```python
from build123d import *

# Parameters (mm, degrees)
SKETCH1_R                = 52.5
BOSS_EXTRUDE1_DEPTH      = 2
SKETCH2_R                = 52.5
SKETCH2_R_2              = 50.25
BOSS_EXTRUDE2_DEPTH      = 100
BOSS_EXTRUDE3_DEPTH      = 90
BOSS_EXTRUDE3_DEPTH_BACK = 15
BOSS_EXTRUDE4_DEPTH      = 15
BOSS_EXTRUDE4_DEPTH_BACK = 10
SKETCH7_R                = 15
SKETCH8_R                = 37.5
BOSS_EXTRUDE5_DEPTH      = 5
SKETCH9_R                = 1.5
CUT_EXTRUDE1_DEPTH       = 6
CUT_EXTRUDE2_DEPTH       = 265.804278799
CUT_EXTRUDE2_DEPTH_BACK  = 265.804278799
SKETCH5_R                = 4.5
CUT_EXTRUDE3_START       = -4
CUT_EXTRUDE3_DEPTH       = 20
CUT_EXTRUDE4_START       = -3
SKETCH11_W               = 8
SKETCH11_H               = 15
CUT_EXTRUDE4_DEPTH       = 95
SKETCH12_R               = 3
CUT_EXTRUDE5_DEPTH       = 20
SKETCH13_R               = 3.5
SKETCH13_R_2             = 3
BOSS_EXTRUDE6_DEPTH      = 6.5
CHAMFER1_SIZE            = 0.5
SKETCH14_R               = 51.5
CUT_EXTRUDE6_DEPTH       = 48
SKETCH15_R               = 1.5
BOSS_EXTRUDE7_DEPTH      = 5
BOSS_EXTRUDE8_DEPTH      = 5
BOSS_EXTRUDE9_DEPTH      = 6
BOSS_EXTRUDE9_DEPTH_BACK = 6
SKETCH18_W               = 4.388119868
SKETCH18_H               = 39.410417959
SKETCH18_W_2             = 3.988119868
SKETCH18_H_2             = 39.010417959
BOSS_EXTRUDE10_DEPTH     = 148
CUT_EXTRUDE7_DEPTH       = 12
CUT_EXTRUDE8_REACH       = 263.976


with BuildPart() as part:
    # Sketch1 → Boss-Extrude1 (new body)
    with BuildSketch(Plane(origin=(0, 0, 0), x_dir=(1, 0, 0), z_dir=(0, 1, 0))):
        with Locations(Location((0, 0, 0), (0, 0, 270))):
            Circle(SKETCH1_R)
    extrude(amount=BOSS_EXTRUDE1_DEPTH)

    # Sketch2 → Boss-Extrude2 (add)
    with BuildSketch(Plane(origin=(0, 2, 0), x_dir=(1, 0, 0), z_dir=(0, 1, 0))):
        with Locations(Location((0, 0, 0), (0, 0, 270))):
            Circle(SKETCH2_R)
        with Locations(Location((0, 0, 0), (0, 0, 270))):
            Circle(SKETCH2_R_2, mode=Mode.SUBTRACT)
    extrude(amount=BOSS_EXTRUDE2_DEPTH)


with BuildPart() as body_2:
    # Sketch6 → Boss-Extrude3 (new, two sides: drawn at the far end of the back side and taken through both)
    with BuildSketch(Plane.XY.offset(-BOSS_EXTRUDE3_DEPTH_BACK)):
        Polygon((32.5, 195), (32.5, 145), (50.5, 106.3), (50.5, 0), (52.5, 0), (62.5, 0), (62.5, 102), (42.5, 145), (42.5, 195), align=None)
    extrude(amount=BOSS_EXTRUDE3_DEPTH + BOSS_EXTRUDE3_DEPTH_BACK)

    # Sketch7 → Boss-Extrude4 (add, two sides: drawn at the far end of the back side and taken through both)
    with BuildSketch(Plane(origin=(42.5, 0, 0), x_dir=(0, 0, -1), z_dir=(1, 0, 0)).offset(-BOSS_EXTRUDE4_DEPTH_BACK)):
        with Locations(Location((0, 180, 0), (0, 0, 90))):
            Circle(SKETCH7_R)
    extrude(amount=BOSS_EXTRUDE4_DEPTH + BOSS_EXTRUDE4_DEPTH_BACK)

    # Sketch8 → Boss-Extrude5 (add)
    with BuildSketch(Plane(origin=(57.5, 0, 0), x_dir=(0, 0, -1), z_dir=(1, 0, 0))):
        with Locations(Location((0, 180, 0), (0, 0, 90))):
            Circle(SKETCH8_R)
    extrude(amount=BOSS_EXTRUDE5_DEPTH)

    # Sketch9 → Cut-Extrude1 (cut)
    with BuildSketch(Plane(origin=(62.5, 0, 0), x_dir=(0, 0, -1), z_dir=(1, 0, 0))):
        with Locations(Location((-35, 180, 0), (0, 0, 90))):
            Circle(SKETCH9_R)
        with Locations(Location((0, 215, 0), (0, 0, 90))):
            Circle(SKETCH9_R)
        with Locations(Location((35, 180, 0), (0, 0, 90))):
            Circle(SKETCH9_R)
        with Locations(Location((0, 145, 0), (0, 0, 90))):
            Circle(SKETCH9_R)
    extrude(amount=-CUT_EXTRUDE1_DEPTH, mode=Mode.SUBTRACT)

    # Sketch5 → Cut-Extrude2 (cut, two sides: drawn at the far end of the back side and taken through both)
    with BuildSketch(Plane(origin=(68.805630826, 0, 0), x_dir=(0, 0, -1), z_dir=(1, 0, 0)).offset(-CUT_EXTRUDE2_DEPTH_BACK)):
        with Locations(Location((0, 180, 0), (0, 0, 90))):
            Circle(SKETCH5_R)
        with Locations(Location((-77, 180, 0), (0, 0, 90))):
            Circle(SKETCH5_R)
    extrude(amount=CUT_EXTRUDE2_DEPTH + CUT_EXTRUDE2_DEPTH_BACK, mode=Mode.SUBTRACT)


with BuildPart() as cut_extrude3_tool:
    # Sketch10 → Cut-Extrude3 (new body)
    with BuildSketch(Plane(origin=(62.5, 0, 0), x_dir=(0, 0, -1), z_dir=(1, 0, 0)).offset(CUT_EXTRUDE3_START)):
        with BuildLine():
            Line((7.5, 2), (-7.5, 2))
            Line((-7.5, 2), (-7.5, 6))
            ThreePointArc((-7.5, 6), (0, 9.309773059), (7.5, 6))
            Line((7.5, 6), (7.5, 2))
        make_face()
    extrude(amount=-CUT_EXTRUDE3_DEPTH)


with BuildPart() as part_1:
    add(part.part)

    # Cut-Extrude3: cut by cut_extrude3_tool
    add(cut_extrude3_tool.part, mode=Mode.SUBTRACT)



with BuildPart() as body_2_1:
    add(body_2.part)

    # Cut-Extrude3: cut by cut_extrude3_tool
    add(cut_extrude3_tool.part, mode=Mode.SUBTRACT)

    # Sketch11 → Cut-Extrude4 (cut)
    with BuildSketch(Plane.XZ.offset(CUT_EXTRUDE4_START)):
        with Locations((56.5, 0)):
            Rectangle(SKETCH11_W, SKETCH11_H)
    extrude(amount=-CUT_EXTRUDE4_DEPTH, mode=Mode.SUBTRACT)

    # Sketch12 → Cut-Extrude5 (cut)
    with BuildSketch(Plane(origin=(0, 0, -15), x_dir=(-1, 0, 0), z_dir=(0, 0, -1))):
        with Locations((-56.5, 93)):
            Circle(SKETCH12_R)
    extrude(amount=-CUT_EXTRUDE5_DEPTH, mode=Mode.SUBTRACT)

    # Sketch13 → Boss-Extrude6 (add)
    with BuildSketch(Plane(origin=(0, 0, -15), x_dir=(-1, 0, 0), z_dir=(0, 0, -1))):
        with Locations(Location((-56.5, 93, 0), (0, 0, 180))):
            Circle(SKETCH13_R)
        with Locations((-56.5, 93)):
            Circle(SKETCH13_R_2, mode=Mode.SUBTRACT)
    extrude(amount=BOSS_EXTRUDE6_DEPTH)

    # Chamfer1
    chamfer1_edges = [body_2_1.edges().sort_by_distance(p)[0] for p in [
        (53, 93, -21.5),
    ]]
    chamfer(chamfer1_edges, length=CHAMFER1_SIZE - 0.0001)  # a hair under: the kernel refuses the full size

    # Sketch14 → Cut-Extrude6 (cut)
    with BuildSketch(Plane(origin=(0, 102, 0), x_dir=(1, 0, 0), z_dir=(0, 1, 0))):
        Circle(SKETCH14_R)
    extrude(amount=CUT_EXTRUDE6_DEPTH, mode=Mode.SUBTRACT)

    # Sketch15 → Boss-Extrude7 (add)
    with BuildSketch(Plane(origin=(62.5, 0, 0), x_dir=(0, 0, -1), z_dir=(1, 0, 0))):
        Polygon((-33.512753614, 163.173076775), (0, 102), (33.512753614, 163.173076775), align=None)
        with Locations(Location((0, 145, 0), (0, 0, 90))):
            Circle(SKETCH15_R, mode=Mode.SUBTRACT)
    extrude(amount=-BOSS_EXTRUDE7_DEPTH)

    # Sketch16 → Boss-Extrude8 (add)
    with BuildSketch(Plane.ZY.offset(-57.5)):
        Polygon((-11.8572367, 170.812729576), (-3.863517383, 104.969648), (3.542835396, 104.969648), (11.646025701, 170.546424731), align=None)
    extrude(amount=BOSS_EXTRUDE8_DEPTH)

    # Sketch17 → Boss-Extrude9 (add, two sides: drawn at the far end of the back side and taken through both)
    with BuildSketch(Plane.XY.offset(-BOSS_EXTRUDE9_DEPTH_BACK)):
        Polygon((44.979042662, 173.247563953), (44.979042662, 165.800390699), (53.161932833, 150.308684598), (53.161932833, 173.247563953), align=None)
    extrude(amount=BOSS_EXTRUDE9_DEPTH + BOSS_EXTRUDE9_DEPTH_BACK)


with BuildPart() as part_2:
    add(part_1.part)

    add(body_2_1.part)  # Boss-Extrude10 merges body 2
    # Sketch18 → Boss-Extrude10 (add)
    with BuildSketch(Plane(origin=(0, 2, 0), x_dir=(1, 0, 0), z_dir=(0, 1, 0))):
        with Locations((37.256595202, -8.286604054)):
            Rectangle(SKETCH18_W, SKETCH18_H)
        with Locations((37.256595202, -8.286604053)):
            Rectangle(SKETCH18_W_2, SKETCH18_H_2, mode=Mode.SUBTRACT)
    extrude(amount=BOSS_EXTRUDE10_DEPTH)

    # Sketch19 → Cut-Extrude7 (cut)
    with BuildSketch(Plane(origin=(62.5, 0, 0), x_dir=(0, 0, -1), z_dir=(1, 0, 0))):
        Polygon((-72.544377907, 13.00185454), (-11.567320289, 13.00185454), (-11.567320289, 53.055277221), (-42.055849098, 111.310144767), (-72.544377907, 53.055277221), align=None)
        Polygon((-76.052706901, 131.115597336), (-44.770106705, 131.115597336), (-60.411406803, 168.245412522), align=None)
        Polygon((-72.544377907, 73.680676562), (-72.544377907, 122.667191379), (-60.262958239, 93.513167119), align=None)
    extrude(amount=-CUT_EXTRUDE7_DEPTH, mode=Mode.SUBTRACT)

    # Cut-Extrude8: up to this face of the body (flat: up to its plane)
    cut_extrude8_end = Plane(part_2.part.faces().sort_by_distance((42.166193849, 124.217683224, 58.964397348))[0])
    # Sketch19<2> → Cut-Extrude8 (cut, up to the picked face)
    with BuildSketch(Plane(origin=(62.5, 0, 0), x_dir=(0, 0, -1), z_dir=(1, 0, 0)), mode=Mode.PRIVATE) as cut_extrude8_sk1:
        Polygon((-72.544377907, 13.00185454), (-11.567320289, 13.00185454), (-11.567320289, 53.055277221), (-42.055849098, 111.310144767), (-72.544377907, 53.055277221), align=None)
    cut_extrude8_tool1 = split(extrude(cut_extrude8_sk1.sketch, amount=-CUT_EXTRUDE8_REACH, mode=Mode.PRIVATE), bisect_by=cut_extrude8_end, keep=Keep.BOTH, mode=Mode.PRIVATE)
    # Sketch19<2> → Cut-Extrude8 (cut, up to the picked face)
    with BuildSketch(Plane(origin=(62.5, 0, 0), x_dir=(0, 0, -1), z_dir=(1, 0, 0)), mode=Mode.PRIVATE) as cut_extrude8_sk2:
        Polygon((-76.052706901, 131.115597336), (-44.770106705, 131.115597336), (-60.411406803, 168.245412522), align=None)
    cut_extrude8_tool2 = split(extrude(cut_extrude8_sk2.sketch, amount=-CUT_EXTRUDE8_REACH, mode=Mode.PRIVATE), bisect_by=cut_extrude8_end, keep=Keep.BOTH, mode=Mode.PRIVATE)
    # Sketch19<2> → Cut-Extrude8 (cut, up to the picked face)
    with BuildSketch(Plane(origin=(62.5, 0, 0), x_dir=(0, 0, -1), z_dir=(1, 0, 0)), mode=Mode.PRIVATE) as cut_extrude8_sk3:
        Polygon((-72.544377907, 73.680676562), (-72.544377907, 122.667191379), (-60.262958239, 93.513167119), align=None)
    cut_extrude8_tool3 = split(extrude(cut_extrude8_sk3.sketch, amount=-CUT_EXTRUDE8_REACH, mode=Mode.PRIVATE), bisect_by=cut_extrude8_end, keep=Keep.BOTH, mode=Mode.PRIVATE)
    add(cut_extrude8_tool1.solids().sort_by(Axis((62.5, 49.636219, 42.055849), (-1, 0, 0)))[0], mode=Mode.SUBTRACT)
    add(cut_extrude8_tool2.solids().sort_by(Axis((62.5, 143.492202, 60.411407), (-1, 0, 0)))[0], mode=Mode.SUBTRACT)
    add(cut_extrude8_tool3.solids().sort_by(Axis((62.5, 96.620345, 68.450571), (-1, 0, 0)))[0], mode=Mode.SUBTRACT)


solid = part_2.part
```
Read the model definition and answer for the solid it produces. Units are mm, in the model's axes. A direction names the side the tool comes from. Coordinates: 2 decimals unless noted, no trailing zeros. Loops run counter-clockwise (first coordinate to the right, second up) from the corner with the lowest first, then second, coordinate; pieces in that order, holes last.
(1) Consider line 1 along X through (y, z) = (134.5, 16); line 2 along X through (y, z) = (78, 0); line 3 along Z through (x, y) = (37.5, 180). Determine where each line is inside the solid, lowest interval first.
Solution:
line 1: x = 35.06 to 35.26, 39.25 to 39.45, 57.5 to 62.5
line 2: x = -52.5 to -50.25, 35.06 to 35.26, 39.25 to 39.45, 50.25 to 52.5, 60.5 to 62.5
line 3: z = -15 to -4.5, 4.5 to 72.5, 81.5 to 90
(2) The mould has two halves that part along X. Classify faces 1 (the face through (37, 75, -11.419)), 2 (the face through (37.43, 184.292, 78.352)): released by +X, released by -X, zero draft, split by the parting line, or undercut.
Solution:
face 1: undercut
face 2: zero draft
(3) The part is cut by section C-C (z = -41.5). Determine the outline of the cut face in (x, y), and give its area (3 significant figures).
Solution:
outline: (-32.16, 0) - (32.16, 0) - (32.16, 102) - (28.33, 102) - (28.33, 2) - (-28.33, 2) - (-28.33, 102) - (-32.16, 102) - close
area: 893 mm2
(4) The part is cut by section B-B (x = 0). Determine the outline of the cut face in (y, z).
Solution:
outline: (0, -52.5) - (102, -52.5) - (102, -50.25) - (2, -50.25) - (2, 50.25) - (102, 50.25) - (102, 52.5) - (0, 52.5) - close
(5) The part is cut by section A-A (y = 85.5). Determine the outline of the cut face in (x, z).
Solution:
outline: (35.06, -11.42) - (39.45, -11.42) - (39.45, 27.99) - (35.06, 27.99) - close; (50.5, -15) - (62.5, -15) - (62.5, 28.55) - (50.5, 28.55) - (50.5, 14.35) arc R52.5 ccw (long way) to (50.5, -14.35) - close; (50.5, 55.56) - (62.5, 55.56) - (62.5, 65.23) - (50.5, 65.23) - close; (50.5, 72.54) - (62.5, 72.54) - (62.5, 90) - (50.5, 90) - close; hole circle Ø100.5 at (0, 0); hole (35.26, -11.22) - (39.25, -11.22) - (39.25, 27.79) - (35.26, 27.79) - close; hole (52.5, -7.5) - (60.5, -7.5) - (60.5, 7.5) - (52.5, 7.5) - close
(6) Flat-ended cylindrical pins translate along their axes: pin 1 Ø10.5 at (y, z) = (180, 0) entering from +X; pin 2 Ø1 at (y, z) = (29, -28.5) entering from +X; pin 3 Ø1.5 at (y, z) = (83.5, -6) entering from -X; pin 4 Ø1 at (y, z) = (37.5, -11) entering from -X. Find the tip coordinate at first contact, or state that the pin passes through.
Solution:
pin 1: stops at x = 62.5
pin 2: stops at x = 44.41
pin 3: stops at x = -52.24
pin 4: stops at x = -51.44
(7) A tool of negligible diameter and unlimited length cuts with its end or side. For faces 3 (the face through (56, 51, -7.5)), 4 (the face through (42.5, 191, -12)), 5 (the face through (37, 173, -15)), from which of +Z, -Z, +X, -X, +Y, -Y can it reach the whole face along a straight path? Write none if from no direction.
Solution:
face 3: none
face 4: -Z, +Y
face 5: -Z, -X, +Y
